Design review of the part built by this model. Coordinates are the model's own, in mm. A direction names the side the tool comes from. Give positions to 0.01 mm unless a question says otherwise; leave off trailing zeros. Write each loop counter-clockwise with the first axis right and the second up, starting at its lowest first coordinate (ties: lowest second). Pieces come first, ordered by that corner, then holes.
```python
from build123d import *

# Parameters (mm, degrees)
BOSS_EXTRUDE1_DEPTH     = 3
SKETCH8_R               = 4
BOSS_EXTRUDE4_DEPTH     = 3
CUT_EXTRUDE5_REACH      = 42.577
SKETCH9_R               = 3.025
CUT_EXTRUDE6_REACH      = 42.577
CUT_EXTRUDE6_END_RADIUS = 4
SKETCH10_R              = 0.8
SKETCH11_R              = 3.5
BOSS_EXTRUDE5_DEPTH     = 4.7
SKETCH12_R              = 2
CUT_EXTRUDE7_DEPTH      = 1.95
SKETCH13_W              = 3
SKETCH13_H              = 7
CUT_EXTRUDE8_DEPTH      = 15


with BuildPart() as part:
    # Sketch3 → Boss-Extrude1 (new body)
    with BuildSketch(Plane.XY):
        Polygon((0, 0), (11.497632607, 6.066666667), (9.670080369, 3.5), (39.670080369, 3.5), (39.670080369, -3.5), (9.670080369, -3.5), (11.497632607, -6.066666667), align=None)
    extrude(amount=BOSS_EXTRUDE1_DEPTH)

    # Sketch8 → Boss-Extrude4 (add)
    with BuildSketch(Plane.XY.offset(3)):
        with Locations(Location((19.835040185, 0, 0), (0, 0, 118.955024372))):
            Circle(SKETCH8_R)
    extrude(amount=BOSS_EXTRUDE4_DEPTH)

    # Sketch9 → Cut-Extrude5 (cut, up to next)
    with BuildSketch(Plane.XY.offset(6), mode=Mode.PRIVATE) as cut_extrude5_sk1:
        with Locations((19.835040185, 0)):
            Circle(SKETCH9_R)
    cut_extrude5_tool1 = extrude(cut_extrude5_sk1.sketch, amount=-CUT_EXTRUDE5_REACH, mode=Mode.PRIVATE) & part.part
    add(cut_extrude5_tool1.solids().sort_by_distance((19.83504, 0, 6))[0], mode=Mode.SUBTRACT)

    # Cut-Extrude6: up to this cylinder (the profile starts inside it)
    cut_extrude6_end = Plane(origin=(19.835040185, 0, 4.5), z_dir=(0, 0, -1)) * Cylinder(CUT_EXTRUDE6_END_RADIUS, 94.154, mode=Mode.PRIVATE)
    # Sketch10 → Cut-Extrude6 (cut, up to the surface)
    with BuildSketch(Plane(origin=(0, 0, 0), x_dir=(1, 0, 0), z_dir=(0, 1, 0)), mode=Mode.PRIVATE) as cut_extrude6_sk1:
        with Locations(Location((19.835040185, -4.5, 0), (0, 0, 270))):
            Circle(SKETCH10_R)
    cut_extrude6_tool1 = extrude(cut_extrude6_sk1.sketch, amount=-CUT_EXTRUDE6_REACH, mode=Mode.PRIVATE) & cut_extrude6_end
    add(cut_extrude6_tool1.solids().sort_by_distance((19.83504, 0, 4.5))[0], mode=Mode.SUBTRACT)

    # Sketch11 → Boss-Extrude5 (add)
    with BuildSketch(Plane(origin=(0, 0, 0), x_dir=(-1, 0, 0), z_dir=(0, 0, -1))):
        with Locations(Location((-19.835040185, 0, 0), (0, 0, 270))):
            Circle(SKETCH11_R)
    extrude(amount=BOSS_EXTRUDE5_DEPTH)

    # Sketch12 → Cut-Extrude7 (cut)
    with BuildSketch(Plane(origin=(0, 0, -4.7), x_dir=(-1, 0, 0), z_dir=(0, 0, -1))):
        with Locations((-19.835040185, 0)):
            Circle(SKETCH12_R)
    extrude(amount=-CUT_EXTRUDE7_DEPTH, mode=Mode.SUBTRACT)

    # Sketch13 → Cut-Extrude8 (cut)
    with BuildSketch(Plane(origin=(39.670080369, 0, 0), x_dir=(0, 0, -1), z_dir=(1, 0, 0))):
        with Locations((-1.5, 0)):
            Rectangle(SKETCH13_W, SKETCH13_H)
    extrude(amount=-CUT_EXTRUDE8_DEPTH, mode=Mode.SUBTRACT)


solid = part.part
```
(1) Consider section D-D, the plane z = -3.75. Give the boundary of the cut face in (x, y), then the cut area to 3 significant figures.
Resolved:
outline: circle Ø7 at (19.84, 0); hole circle Ø4 at (19.84, 0)
area: 25.9 mm2
(2) Consider section B-B, the plane y = -0.25. Give the boundary of the cut face in (x, z).
Resolved:
outline: (0.47, 0) - (16.34, 0) - (16.34, -4.7) - (17.85, -4.7) - (17.85, -2.75) - (21.82, -2.75) - (21.82, -4.7) - (23.33, -4.7) - (23.33, 0) - (24.67, 0) - (24.67, 3) - (23.83, 3) - (23.83, 6) - (22.85, 6) - (22.85, 0) - (16.82, 0) - (16.82, 6) - (15.84, 6) - (15.84, 3) - (0.47, 3) - close
(3) Mouldability with a two-part tool opening along Y and no side actions: class faces 4 (the face through (20, 0, -2.75)), 5 (the face through (5.67, 2.99, 1.48)), 6 (the face through (5.829, -3.076, 1.479)) as pulls with the +Y half, pulls with the -Y half, needs draft (parallel to the pull), parting line crosses it, or undercut.
Resolved:
face 4: undercut
face 5: pulls with the +Y half
face 6: pulls with the -Y half
(4) To check wall thickness, follow L1, parallel to Y at x = 19.75, z = 0.25; L2, parallel to Z at x = 3.75, y = 0; L3, parallel to X at y = -3.15, z = 4.5. State the ranges of each line that lie inside material, in increasing order.
Resolved:
L1: y = -3.5 to -3.02, 3.02 to 3.5
L2: z = 0 to 3
L3: x = 17.37 to 19.04, 20.64 to 22.3
(5) Consider section C-C, the plane x = 12.5. Give the boundary of the cut face in (y, z), then the cut area to 3 significant figures.
Resolved:
outline: (-3.5, 0) - (3.5, 0) - (3.5, 3) - (-3.5, 3) - close
area: 21.0 mm2
(6) Consider section A-A, the plane z = 0.25. Give the boundary of the cut face in (x, y) (3 decimals), then the cut area to 3 significant figures.
Resolved:
outline: (0, 0) - (11.498, -6.067) - (9.67, -3.5) - (24.67, -3.5) - (24.67, 3.5) - (9.67, 3.5) - (11.498, 6.067) - close; hole circle Ø6.05 at (19.835, 0)
area: 129 mm2
(7) Clearance check with flat-ended pins moving along their axes: P1, Ø3, axis at x = 19.84, y = 0, coming from the -Z side; P2, Ø3, axis at x = 19, y = -1, coming from the +Z side; P3, Ø3, axis at y = 1, z = -3, coming from the +X side. State where each tip first meets the part, or that it passes through.
Resolved:
P1: stops at z = -2.75
P2: stops at z = 0
P3: stops at x = 23.34
(8) Tool access review of faces 1 (the face through (24, 0, 3)), 2 (the face through (16.365, 0.456, -2.317)), 3 (the face through (20, 0, 0)): name each direction out of +Z, -Z, +X, -X, +Y, -Y from which nothing blocks a thin tool from reaching the whole face with its end or side.
Resolved:
face 1: +Z, +X
face 2: -Z
face 3: +Z
